Autodesk Inventor part; units mm, degrees
ref_plane "body_screw_XY" through (0, -7, 3) normal (0, 0, 1) x (1, 0, 0)
ref_plane "body_screw_YZ" through (0, -7, 3) normal (1, 0, 0) x (0, 1, 0)
ref_plane "body_screw_ZX" through (0, -7, 3) normal (0, 1, 0) x (0, 0, 1)
sketch "Sketch_1" plane through (0, 0, 0) normal (0, 0, 1) x (1, 0, 0)
  line L0 (3, 0) -> (-3, 0)
  line L1 (-3, 10.5) -> (-3, 4.5)
  line L2 (-3, 4.5) -> (-2.5, 4)
  line L3 (-2.5, 4) -> (2.5, 4)
  line L4 (2.5, 4) -> (3, 4.5)
  line L5 (3, 4.5) -> (3, 10.5)
  line L6 (3, 10.5) -> (2.5, 11)
  line L7 (2.5, 11) -> (-2.5, 11)
  line L8 (-2.5, 11) -> (-3, 10.5)
revolve "Revolution1" add sketch "Sketch_1" angle 360 about axis through (3, 0, 0) along (1, 0, 0)
sketch "Sketch_2" plane through (0, 0, 0) normal (1, 0, 0) x (0, 1, 0)
  line L0 (-11, 0.75) -> (-11, -0.75)
  line L1 (-11, -0.75) -> (9, -0.75)
  line L2 (9, -0.75) -> (9, 0.75)
  line L3 (9, 0.75) -> (-11, 0.75)
extrude "Extrusion1" cut sketch "Sketch_2" along normal mid plane 6
sketch "Sketch_3" plane through (0, 0, 0) normal (1, 0, 0) x (0, 1, 0)
  line L0 (-7, 11) -> (-7, 0)
  line L1 (-7, 0) -> (-8.45, 0)
  line L2 (-8.45, 0) -> (-8.45, 3)
  line L3 (-8.45, 3) -> (-9.45, 3)
  line L4 (-9.45, 3) -> (-9.45, 11)
  line L5 (-9.45, 11) -> (-7, 11)
  line L6 (-7, 11) -> (-7, 0)
revolve "Revolution2" cut sketch "Sketch_3" angle 360 about axis through (0, -7, 11) along (0, 0, 1)
sketch "Sketch_4" plane through (0, 0, 0) normal (1, 0, 0) x (0, 1, 0)
  line L0 (-7, -11.25) -> (-7, -0.75)
  line L1 (-7, -0.75) -> (-5.75, -0.75)
  line L2 (-5.75, -0.75) -> (-5.9935, -0.9935)
  line L3 (-5.9935, -0.9935) -> (-5.9935, -11.25)
  line L4 (-5.9935, -11.25) -> (-7, -11.25)
  line L5 (-7, -11.25) -> (-7, -0.75)
revolve "Revolution3" cut sketch "Sketch_4" angle 360 about axis through (0, -7, -11.25) along (0, 0, -1)
thread "Thread1"
sketch "Sketch_7" plane through (0, 0, -7.5) normal (0, 0, 1) x (1, 0, 0)
  line L0 (3, 0) -> (-3, 0)
  line L1 (-3, 0) -> (-3, 1.5)
  line L2 (-3, 1.5) -> (-2.7295, 1.2295)
  line L3 (-2.7295, 1.2295) -> (2.7295, 1.2295)
  line L4 (2.7295, 1.2295) -> (3, 1.5)
  line L5 (3, 1.5) -> (3, 0)
  line L6 (3, 0) -> (-3, 0)
revolve "Revolution4" cut sketch "Sketch_7" angle 360 about axis through (3, 0, -7.5) along (1, 0, 0)
thread "Thread2"
sketch "Sketch_8" plane through (0, 0, 7.5) normal (0, 0, 1) x (1, 0, 0)
  line L0 (3, 0) -> (-3, 0)
  line L1 (-3, 0) -> (-3, 1.5)
  line L2 (-3, 1.5) -> (-2.7295, 1.2295)
  line L3 (-2.7295, 1.2295) -> (2.7295, 1.2295)
  line L4 (2.7295, 1.2295) -> (3, 1.5)
  line L5 (3, 1.5) -> (3, 0)
  line L6 (3, 0) -> (-3, 0)
revolve "Revolution5" cut sketch "Sketch_8" angle 360 about axis through (3, 0, 7.5) along (1, 0, 0)
thread "Thread3"
ref_plane "body_screw_XY" through (0, -7, 3) normal (0, 0, 1) x (1, 0, 0)
ref_plane "body_screw_YZ" through (0, -7, 3) normal (1, 0, 0) x (0, 1, 0)
ref_plane "body_screw_ZX" through (0, -7, 3) normal (0, 1, 0) x (0, 0, 1)
properties part number "SCSWJ8-6_b"
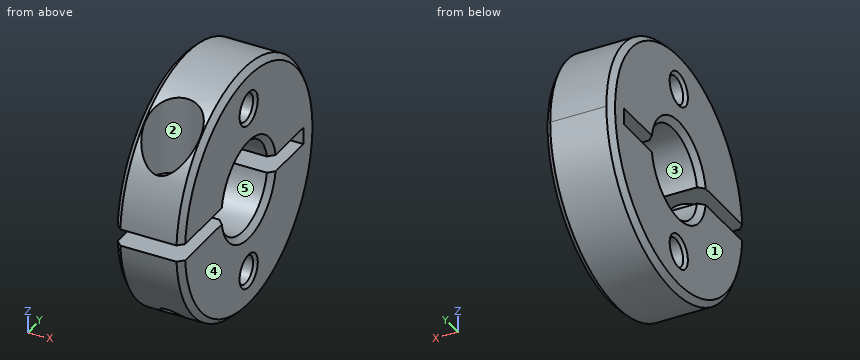
Part model, mm, in its own coordinate system. Face numbers are marked on the shaded views. A direction names the side the tool comes from. Coordinates: 2 decimals unless noted, no trailing zeros. Write each loop counter-clockwise with the first axis right and the second up, starting at its lowest first coordinate (ties: lowest second). Pieces come first, ordered by that corner, then holes.
Item 1: Mould opens along Z. For the marked faces 3, 4 and 5 say: released by +Z, released by -Z, zero draft, split by the parting line, or undercut.
Item 2: Pin check, flat tips, straight feed: pin 1 (1.6 mm diameter, centred on x = 0, y = -7, fed in from -Z); pin 2 (4 mm diameter, centred on y = 0, z = -7.5, fed in from +X); pin 3 (2 mm diameter, centred on x = 2.5, y = 5, fed in from +Z); pin 4 (1.5 mm diameter, centred on x = -1, y = 5, fed in from -Z). Stop position of each tip, or through.
Item 3: Slice it at B-B (x = 0). Write the cut outline in (y, z).
Item 4: Slice it at A-A (y = 0). Count the separate pieces of the cut face and the enclosed holes in it, and give its area (3 significant figures).
Item 5: Probe line 1 (X direction, y = -7, z = 5); line 2 (Z direction, x = -1.25, y = 0); line 3 (Z direction, x = 0.25, y = 7.5). List the from-to ranges inside material, lowest first.
Item 6: Which spindle directions (+Z, -Z, +X, -X, +Y, -Y) get a long thin tool onto all of the face, cutting with end or side? Do the marked faces 1 and 2. Say none if no direction does.
Results found:
1. face 3: undercut
1. face 4: zero draft
1. face 5: undercut
2. pin 1: passes through
2. pin 2: stops at x = 3
2. pin 3: stops at z = 10.25
2. pin 4: stops at z = -10.15
3. outline: (-10.97, -0.75) arc R11 ccw to (-8.01, -7.54) - (-8.01, -0.99) - (-8.25, -0.75) - close; (-10.97, 0.75) - (-8.45, 0.75) - (-8.45, 3) - (-9.45, 3) - (-9.45, 5.63) arc R11 ccw to start; (-5.99, -9.22) arc R11 ccw (long way) to (-4.55, 10.01) - (-4.55, 3) - (-5.55, 3) - (-5.55, 0.75) - (-3.93, 0.75) arc R4 cw to (3.93, 0.75) - (9, 0.75) - (9, -0.75) - (3.93, -0.75) arc R4 cw to (-3.93, -0.75) - (-5.75, -0.75) - (-5.99, -0.99) - close; hole circle Ø2.46 at (0, -7.5); hole circle Ø2.46 at (0, 7.5)
4. separate pieces: 4
4. enclosed holes: 0
4. area: 53.2 mm2
5. line 1: x = -3 to -2.45, 2.45 to 3
5. line 2: z = -11 to -8.73, -6.27 to -4, 4 to 6.27, 8.73 to 11
5. line 3: z = -8.05 to -0.75, 0.75 to 8.05
6. face 1: +Z, -Z, -X, +Y, -Y
6. face 2: +Z
